Source: CAD feature listing. Evaluate the final solid. Frame: model axes, mm. Coordinates: 2 decimals unless noted, no trailing zeros. Order: outer loops, then holes, each group sorted by start corner. A loop starts at its lowest first (then second) coordinate and runs counter-clockwise, first axis right, second up.
Item 1: Section C-C on x = 364. Return the cut outline in (y, z).
Item 2: Ray query, line 1 (X direction, y = 36, z = 0.4); line 2 (X direction, y = 35.5, z = 1.35); line 3 (Y direction, x = 365, z = 1.65). Return the intervals inside material, ascending.
Item 3: Section A-A on x = 205.5. Return the cut outline in (y, z), then the cut area to 3 significant figures.
Item 4: Contact query for flat-ended pins moving along their axis: P1, Ø3, axis at x = 265.73, y = 18.28, coming from the +Z side; P2, Ø1, axis at x = 361, z = 1.5, coming from the -Y side; P3, Ø1, axis at x = 277, z = 0.5, coming from the -Y side. Output: stop coordinate, or through.
Item 5: Section B-B on z = 1.4. State how many separate pieces and enclosed holes the cut face has, then the cut area to 3 significant figures.
Item 6: Section D-D on x = 297. Return the cut outline in (y, z), then the cut area to 3 significant figures.
from build123d import *

# Parameters (mm, degrees)
EXTRUDE_1_DEPTH     = 3
CUT_EXTRUDE_2_DEPTH = 10
SKETCH1_R           = 1.5
SKETCH1_R_2         = 1.6
CUT_EXTRUDE2_DEPTH  = 3
CHAMFER1_SIZE       = 10
SKETCH2_R           = 1.6
CUT_EXTRUDE3_DEPTH  = 10
SKETCH3_R           = 1.6
CUT_EXTRUDE4_DEPTH  = 39


with BuildPart() as part:
    # 草图1 → 凸台-拉伸1 (new body)
    with BuildSketch(Plane.XY):
        Polygon((-31.770103996, 71.767703031), (408.229896004, 71.767703031), (408.229896004, -16.727308921), (-31.770103996, 21.767703031), align=None)
    extrude(amount=EXTRUDE_1_DEPTH)

    # 草图3 → 切除-拉伸2 (cut)
    with BuildSketch(Plane.XY.offset(3)):
        Polygon((0.108126343, 18.978719263), (0.369593572, 21.967303357), (-31.770103996, 24.779162543), (-31.770103996, 21.767703031), align=None)
        Polygon((371.792330274, -7.315752), (371.496000749, -10.702813974), (341.211681927, -8.053279394), (341.508011452, -4.666217421), align=None)
        Polygon((217.38215207, 6.193388126), (217.085822544, 2.806326152), (186.801503722, 5.455860732), (187.097833248, 8.842922705), align=None)
        Polygon((62.971973866, 19.702528252), (62.67564434, 16.315466278), (32.391325518, 18.965000858), (32.687655044, 22.352062831), align=None)
    extrude(amount=-CUT_EXTRUDE_2_DEPTH, mode=Mode.SUBTRACT)

    # Sketch1 → Cut-Extrude2 (cut)
    with BuildSketch(Plane(origin=(0, 0, 0), x_dir=(-1, 0, 0), z_dir=(0, 0, -1))):
        with Locations((22.792159026, 44.070090887)):
            Circle(SKETCH1_R)
        with Locations((2.868265064, 42.326976033)):
            Circle(SKETCH1_R)
        with Locations((-230.729896004, 56.783526399)):
            Circle(SKETCH1_R_2)
        with Locations((-230.729896004, 18.2779729)):
            Circle(SKETCH1_R_2)
        with Locations((-265.729896004, 18.2779729)):
            Circle(SKETCH1_R_2)
        with Locations((-265.729896004, 56.783526399)):
            Circle(SKETCH1_R_2)
    extrude(amount=-CUT_EXTRUDE2_DEPTH, mode=Mode.SUBTRACT)

    # Chamfer1
    chamfer1_edges = [part.edges().sort_by_distance(p)[0] for p in [
        (-31.770103996, 71.767703031, 1.5),
        (408.229896004, 71.767703031, 1.5),
    ]]
    chamfer(chamfer1_edges, length=CHAMFER1_SIZE)

    # Sketch2 → Cut-Extrude3 (cut)
    with BuildSketch(Plane(origin=(0, 0, 0), x_dir=(-1, 0, 0), z_dir=(0, 0, -1))):
        with Locations((-390.440589081, 36.023865482)):
            Circle(SKETCH2_R)
        with Locations((-387.825916798, 6.138024539)):
            Circle(SKETCH2_R)
    extrude(amount=-CUT_EXTRUDE3_DEPTH, mode=Mode.SUBTRACT)

    # Sketch3 → Cut-Extrude4 (cut)
    with BuildSketch(Plane(origin=(0, 0, 0), x_dir=(-1, 0, 0), z_dir=(0, 0, -1))):
        with Locations((-390.440589081, 56.023865482)):
            Circle(SKETCH3_R)
        with Locations((-14.229896004, 36.023865482)):
            Circle(SKETCH3_R)
        with Locations((-14.229896004, 56.023865482)):
            Circle(SKETCH3_R)
    extrude(amount=-CUT_EXTRUDE4_DEPTH, mode=Mode.SUBTRACT)


solid = part.part
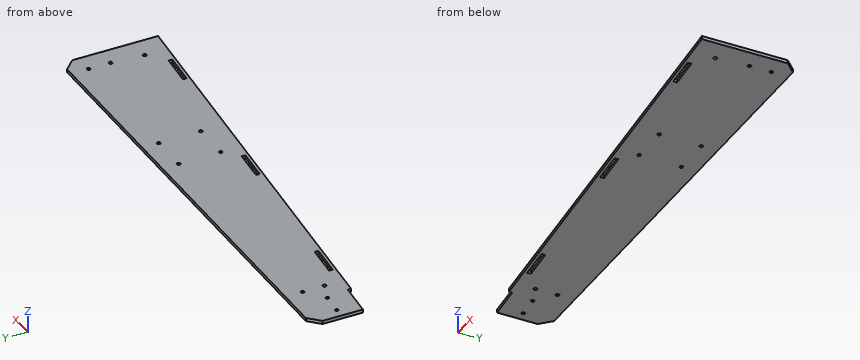
Answer list:
1. outline: (-12.86, 0) - (-10.05, 0) - (-10.05, 3) - (-12.86, 3) - close; (-6.63, 0) - (71.77, 0) - (71.77, 3) - (-6.63, 3) - close
2. line 1: x = -31.77 to 12.63, 15.83 to 388.84, 392.04 to 408.23
2. line 2: x = -31.77 to 12.72, 15.74 to 388.93, 391.95 to 408.23
2. line 3: y = -12.95 to -10.13, -6.72 to 71.77
3. outline: (1.01, 0) - (3.82, 0) - (3.82, 3) - (1.01, 3) - close; (7.23, 0) - (71.77, 0) - (71.77, 3) - (7.23, 3) - close
3. area: 202 mm2
4. P1: passes through
4. P2: stops at y = -12.64
4. P3: stops at y = -5.29
5. separate pieces: 1
5. enclosed holes: 14
5. area: 29,900 mm2
6. outline: (-7, 0) - (71.77, 0) - (71.77, 3) - (-7, 3) - close
6. area: 236 mm2
